from build123d import *

# Parameters (mm, degrees)
F0_W     = 22
F0_H     = 33
F0_R     = 1.1
F1_DEPTH = 1.5
F2_R     = 1.1
F3_DEPTH = 1.5
F4_R     = 1


# Not quite as in the source:
# - a feature names something its author has since deleted; it is built from what else it names


with BuildPart() as f1:
    # F0 (on Top) → F1 (new body)
    with BuildSketch(Plane.XY):
        Rectangle(F0_W, F0_H)
        with Locations((-8, 13.5)):
            Circle(F0_R, mode=Mode.SUBTRACT)
        with Locations((8, 13.5)):
            Circle(F0_R, mode=Mode.SUBTRACT)
    extrude(amount=F1_DEPTH)

    # F2 (on face) → F3 (cut, through all)
    with BuildSketch(Plane.XY.offset(1.5)):
        with BuildLine():
            Line((4, 10), (-4, 10))
            ThreePointArc((-4, 10), (-4.7071067812, 9.7071067812), (-5, 9))
            Line((-5, 9), (-5, 8))
            ThreePointArc((-5, 8), (-4.7071067812, 7.2928932188), (-4, 7))
            Line((-4, 7), (4, 7))
            ThreePointArc((4, 7), (4.7071067812, 7.2928932188), (5, 8))
            Line((5, 8), (5, 9))
            ThreePointArc((5, 9), (4.7071067812, 9.7071067812), (4, 10))
        make_face()
        with BuildLine():
            Line((4, 1), (-4, 1))
            ThreePointArc((-4, 1), (-4.7071067812, 0.7071067812), (-5, 0))
            Line((-5, 0), (-5, -1))
            ThreePointArc((-5, -1), (-4.7071067812, -1.7071067812), (-4, -2))
            Line((-4, -2), (4, -2))
            ThreePointArc((4, -2), (4.7071067812, -1.7071067812), (5, -1))
            Line((5, -1), (5, 0))
            ThreePointArc((5, 0), (4.7071067812, 0.7071067812), (4, 1))
        make_face()
        Polygon((11, -16.5), (11, 0), (-3, -16.5), align=None)
        with Locations((-8, 4)):
            Circle(F2_R)
        with Locations((-8, -11)):
            Circle(F2_R)
    extrude(amount=-F3_DEPTH, mode=Mode.SUBTRACT)

    # F4
    f4_edges = [f1.edges().sort_by_distance(p)[0] for p in [
        (-11, 16.5, 0.75),
        (11, 16.5, 0.75),
        (-11, -16.5, 0.75),
        (11, 0, 0.75),
        (-3, -16.5, 0.75),
    ]]
    fillet(f4_edges, radius=F4_R)


solid = f1.part
For this review, take the finished solid that the model builds, in its own axes (mm). A direction names the side the tool comes from. Give positions to 0.01 mm unless a question says otherwise; leave off trailing zeros. Loops run counter-clockwise (first coordinate to the right, second up) from the corner with the lowest first, then second, coordinate; pieces in that order, holes last. Notation, with made-up numbers: M 63.5,31 L 79.5,31 A8 cw 79.5,44 Z; hole C 80.25,-2 d6. An arc over 180 degrees is marked long. Answer as a JSON object with one key per item and string values. Group by question number.
Q1. Add section A-A on x = -8. Give the boundary of the cut face in (y, z), and give its area (3 significant figures).
Q2. For probe 1 along Y at (x, z) = (-8, 1.2); probe 2 along Y at (x, z) = (4.25, 0.7); probe 3 along Y at (x, z) = (0.25, 1.35), list the stretches that pass through material, from the lowest coordinate up. Write a range as [from, to].
Q3. Add section D-D on y = 4. Give the boundary of the cut face in (x, z).
Q4. Add section C-C on z = 0.9. Give the number of separate pieces and of enclosed holes in the cut face, and give its area (3 significant figures).
Q5. Add section B-B on y = 13.5. Give the boundary of the cut face in (x, z), and give its area (3 significant figures).
Q6. Mouldability with a two-part tool opening along X and no side actions: class faces 3 (the flat face through (0, 1, 1)), 4 (the cylindrical face through (4.715, 9.699, 0.76)), 5 (the flat face through (-11, 0, 1)), 6 (the cylindrical face through (10.699, 16.215, 0.76)) as +X half, -X half, draft (parallel to the pull), parting line (faces both ways), or undercut.
Q7. Tool access review of faces 1 (the flat face through (0, 4, 1.5)), 2 (the cylindrical face through (4.699, -1.715, 0.76)): name each direction out of +Z, -Z, +X, -X, +Y, -Y from which nothing blocks a thin tool from reaching the whole face with its end or side.
Checked values:
{
 "1": {"outline": "M -16.5,0 L -12.1,0 L -12.1,1.5 L -16.5,1.5 Z; M -9.9,0 L 2.9,0 L 2.9,1.5 L -9.9,1.5 Z; M 5.1,0 L 12.4,0 L 12.4,1.5 L 5.1,1.5 Z; M 14.6,0 L 16.5,0 L 16.5,1.5 L 14.6,1.5 Z", "area": "39.6 mm²"},
 "2": {"probe 1": "[-16.5, -12.1], [-9.9, 2.9], [5.1, 12.4], [14.6, 16.5]", "probe 2": "[-7.96, -1.97], [0.97, 7.03], [9.97, 16.5]", "probe 3": "[-12.67, -2], [1, 7], [10, 16.5]"},
 "3": {"outline": "M -11,0 L -9.1,0 L -9.1,1.5 L -11,1.5 Z; M -6.9,0 L 11,0 L 11,1.5 L -6.9,1.5 Z"},
 "4": {"separate pieces": "1", "enclosed holes": "6", "area": "536 mm²"},
 "5": {"outline": "M -11,0 L -9.1,0 L -9.1,1.5 L -11,1.5 Z; M -6.9,0 L 6.9,0 L 6.9,1.5 L -6.9,1.5 Z; M 9.1,0 L 11,0 L 11,1.5 L 9.1,1.5 Z", "area": "26.4 mm²"},
 "6": {"face 3": "undercut", "face 4": "undercut", "face 5": "-X half", "face 6": "+X half"},
 "7": {"face 1": "+Z, +X, -X, +Y, -Y", "face 2": "+Z, -Z"}
}
